Here's how the part is built. I have some questions about the finished solid (model axes, mm). Give positions to 0.01 mm unless a question says otherwise; leave off trailing zeros. Write each loop counter-clockwise with the first axis right and the second up, starting at its lowest first coordinate (ties: lowest second). Pieces come first, ordered by that corner, then holes. Notation, with made-up numbers: (5, -11) - (38, -11) arc R20 ccw to (38, 12) - close; hole circle Ø5 at (78.25, 78). An arc over 180 degrees is marked (long way). Use one line per item in the form item = value. Start each with the question number.
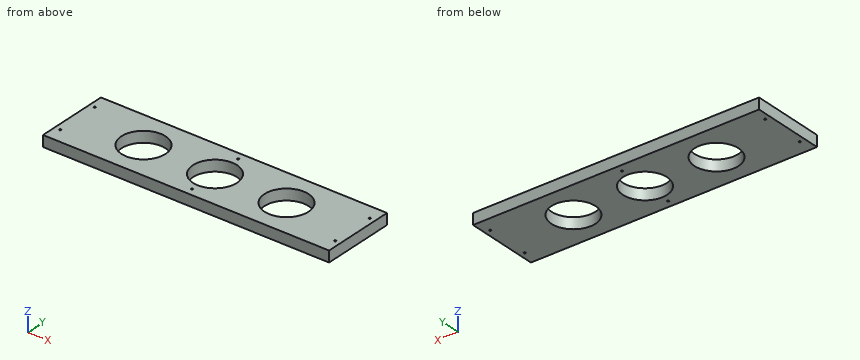
from build123d import *

# Parameters (mm, degrees)
SKETCH1_W           = 495.046
SKETCH1_H           = 127
BOSS_EXTRUDE1_DEPTH = 19.05
SKETCH2_R           = 38.1
CUT_EXTRUDE1_DEPTH  = 5423.392257673
HOLE1_D             = 3.175
HOLE1_DEPTH         = 50.8
HOLE1_CSINK_D       = 10.16
HOLE1_CSINK_ANGLE   = 82
HOLE1_TIP           = 0.953866233


with BuildPart() as part:
    # Sketch1 → Boss-Extrude1 (new body)
    with BuildSketch(Plane.XY):
        with Locations((90.196398512, 5348.331529292)):
            Rectangle(SKETCH1_W, SKETCH1_H)
    extrude(amount=BOSS_EXTRUDE1_DEPTH)

    # Sketch2 → Cut-Extrude1 (cut, through all)
    with BuildSketch(Plane(origin=(0, 0, 0), x_dir=(-1, 0, 0), z_dir=(0, 0, -1))):
        with Locations((-213.957898512, 5348.331529292)):
            Circle(SKETCH2_R)
        with Locations((-90.196398512, 5348.331529292)):
            Circle(SKETCH2_R)
        with Locations((33.565101488, 5348.331529292)):
            Circle(SKETCH2_R)
    extrude(amount=-CUT_EXTRUDE1_DEPTH, mode=Mode.SUBTRACT)

    # Hole1
    with Locations(Plane(origin=(90.196398512, 2347.321529292, 38.1), x_dir=(1, 0, 0), z_dir=(0, 0, 1))):
        with Locations((0, 2696.21), (-237.998, 3089.91), (-237.998, 3039.11), (-237.998, 2962.91), (-237.998, 2912.11), (-237.998, 2835.91), (-237.998, 2785.11), (-237.998, 2708.91), (237.998, 2708.91), (237.998, 2785.11), (237.998, 2835.91), (237.998, 2912.11), (237.998, 2962.91), (237.998, 3039.11), (237.998, 3089.91), (0, 3051.81), (0, 2950.21), (0, 2797.81)):
            CounterSinkHole(HOLE1_D / 2, HOLE1_CSINK_D / 2, depth=HOLE1_DEPTH, counter_sink_angle=HOLE1_CSINK_ANGLE)
            with Locations((0, 0, -(HOLE1_DEPTH + HOLE1_TIP / 2))):  # 118° drill point
                Cone(0, HOLE1_D / 2, HOLE1_TIP, mode=Mode.SUBTRACT)


solid = part.part
1. Please list where these lines run through material, in increasing order: line 1 (X direction, y = 5310, z = 9.5); line 2 (X direction, y = 5318, z = 15.5); line 3 (X direction, y = 5367, z = 12.5).
2. I want a section at C-C, the plane z = 5.25. Give the number of separate pieces and of enclosed holes in the cut face, then the cut area to 3 significant figures.
3. I want a section at B-B, the plane x = -65.5. List the corners of the cut face in (y, z) for me.
4. I want a section at D-D, the plane x = 115. List the corners of the cut face in (y, z) for me, then the cut area to 3 significant figures.
5. I want a section at A-A, the plane y = 5319.5. List the corners of the cut face in (x, z) for me, then the cut area to 3 significant figures.
Result sheet:
q1.line_1 = -157.33 to -149.37, -146.23 to 326.62, 329.76 to 337.72
q1.line_2 = -157.33 to -56.62, -10.51 to 67.14, 113.25 to 190.9, 237.01 to 337.72
q1.line_3 = -157.33 to -66.78, -0.35 to 56.98, 123.41 to 180.74, 247.17 to 337.72
q2.separate_pieces = 1
q2.enclosed_holes = 9
q2.area = 49,100 mm2
q3.outline = (5284.83, 0) - (5327.55, 0) - (5327.55, 19.05) - (5284.83, 19.05) - close; (5369.11, 0) - (5411.83, 0) - (5411.83, 19.05) - (5369.11, 19.05) - close
q4.outline = (5284.83, 0) - (5319.41, 0) - (5319.41, 19.05) - (5284.83, 19.05) - close; (5377.25, 0) - (5411.83, 0) - (5411.83, 19.05) - (5377.25, 19.05) - close
q4.area = 1,320 mm2
q5.outline = (-157.33, 0) - (-58.47, 0) - (-58.47, 19.05) - (-157.33, 19.05) - close; (-8.66, 0) - (65.29, 0) - (65.29, 19.05) - (-8.66, 19.05) - close; (115.1, 0) - (189.05, 0) - (189.05, 19.05) - (115.1, 19.05) - close; (238.86, 0) - (337.72, 0) - (337.72, 19.05) - (238.86, 19.05) - close
q5.area = 6,580 mm2
